Autodesk Inventor part; units mm, degrees
ref_plane "Work Plane1" through (60, 0, 0) normal (0, 0, 1) x (1, 0, 0)
ref_plane "YZ Plane" through (0, 0, 0) normal (1, 0, 0) x (0, 1, 0)
ref_plane "XZ Plane" through (0, 0, 0) normal (0, 1, 0) x (-1, 0, 0)
sketch "Sketch1" plane through (0, 0, 0) normal (0, 0, 1) x (1, 0, 0)
  line L0 (0, 3.175) -> (22.225, 3.175)
  line L1 (22.225, 3.175) -> (22.225, 0)
  line L2 (22.225, 0) -> (0, 0)
  line L3 (-4.445, 0) -> (26.67, 0)
  line L4 (0, -0.635) -> (0, 3.81)
  line L5 (0, 3.175) -> (0, 0)
  dimension "d1" = 6.35
  dimension "d52" = 22.225
revolve "Body" add sketch "Sketch1" angle 360 about axis through (22.225, 0, 0) along (-1, 0, 0)
sketch "Sketch2" plane through (0, 0, 0) normal (-1, 0, 0) x (0, 0, 1)
  line L0 (0, 5.4993) -> (4.7625, 2.7496)
  line L1 (4.7625, 2.7496) -> (4.7625, -2.7496)
  line L2 (4.7625, -2.7496) -> (0, -5.4993)
  line L3 (0, -5.4993) -> (-4.7625, -2.7496)
  line L4 (-4.7625, -2.7496) -> (-4.7625, 2.7496)
  line L5 (-4.7625, 2.7496) -> (0, 5.4993)
  line L6 (-6.6675, 0) -> (6.6675, 0)
  line L7 (0, 7.699) -> (0, -7.699)
  point P0 (0, 0)
  point P1 (0, 0)
  dimension "d10" = 9.525
extrude "Head" add sketch "Sketch2" along normal blind 4.826
sketch "Sketch3" plane through (0, 0, 0) normal (0, 0, 1) x (1, 0, 0)
  line L0 (-4.826, 0.9525) -> (-2.2606, 0.9525)
  line L1 (-2.2606, 0.9525) -> (-2.2606, -0.9525)
  line L2 (-2.2606, -0.9525) -> (-4.826, -0.9525)
  line L3 (-4.826, -0.9525) -> (-4.826, 0.9525)
  line L4 (-2.2606, 0) -> (-4.826, 0) construction
  line L5 (-5.3391, 0) -> (-1.7475, 0)
  line L6 (-4.826, 2.7496) -> (-4.826, -2.7496)
  dimension "d11" = 1.905
  dimension "d13" = 2.5654
extrude "Slot" cut sketch "Sketch3" along normal through all both and the other way through all
sketch "Sketch4" plane through (0, 0, 0) normal (0, 0, 1) x (1, 0, 0)
  line L0 (-4.826, 4.7625) -> (-4.826, 5.4993)
  line L1 (-4.826, 5.4993) -> (-4.4006, 5.4993)
  line L2 (-4.4006, 5.4993) -> (-4.826, 4.7625)
  line L3 (-4.4006, 5.4993) -> (-4.826, 5.4993)
  line L4 (-4.826, 5.4993) -> (-4.826, 4.7625)
  line L5 (-4.826, 5.4993) -> (-4.826, 2.7496)
  line L6 (-5.7912, 0) -> (0.9652, 0)
  line L7 (0, 5.4993) -> (-4.826, 5.4993)
  dimension "d4" = 30
  dimension "d17" = 9.525
revolve "Chamfer1" cut sketch "Sketch4" angle 360 about axis through (-10, 0, 0) along (1, 0, 0)
thread "Thread"
chamfer "Chamfer2" distance 0.635 distance2 0.6351 1 edges at (22.225, -3.175, 0) measured on face at (22.225, -0.1276, -1.0506)
ref_plane "Work Plane1" through (60, 0, 0) normal (0, 0, 1) x (1, 0, 0)
equation "\"d1\" = GD"
equation "\"d52\" = NLG"
equation "\"d10\" = SW"
equation "\"d2\" = KOH - SD"
equation "\"d11\" = SBR"
equation "\"d13\" = STI"
equation "\"d4\" = ANG1"
equation "\"d17\" = SW0"
equation "\"d15\" = GEL"
equation "\"d5\" = -0.5 * SPD + 0.5 * GD"
equation "\"NLG\" = 22.225"
equation "\"GD\" = NND"
equation "\"KOH\" = 4.826"
equation "\"GEL\" = 19.05"
equation "\"SW\" = 9.525"
equation "\"SW0\" = 9.525"
equation "\"SPD\" = GD1"
equation "\"SD2\" = NND"
equation "\"SD\" = 0"
equation "\"ANG1\" = 30deg"
equation "\"GUL\" = -0.5 * GD1 + 0.5 * NND"
equation "\"STI\" = 2.5654"
equation "\"SBR\" = 1.905"
equation "\"RR\" = 0.57912"
equation "\"THREADDIA\" = 6.35"
equation "\"TOA\" = 30deg"
equation "\"BDM\" = NND"
equation "\"FAWI\" = 45deg"
equation "\"NND\" = 6.35"
equation "\"E0\" = 1.155 * SW"
equation "\"GAL\" = 0.635"
equation "\"GD1\" = 5.08"
properties part number "ANSI B18.6.3 - 1/4-20x0.875, SHHMSI" material "Steel, Mild"
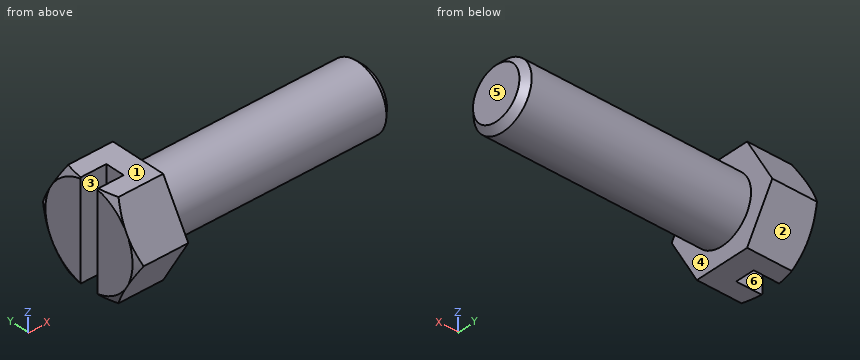
Work out the finished part from the listing and answer in its coordinate system (mm). Face numbers are marked on the shaded views. A direction names the side the tool comes from. Give positions to 0.01 mm unless a question says otherwise; leave off trailing zeros. Loops run counter-clockwise (first coordinate to the right, second up) from the corner with the lowest first, then second, coordinate; pieces in that order, holes last. Notation, with made-up numbers: (-33.75, -4.75) -> (-5.75, -4.75) arc R25 cw to (-5.75, 33.25) -> close; hole circle Ø10 at (-7.75, 29.5). An arc over 180 degrees is marked (long way). Use a Markdown table: item, result. Add a question column.
1. Determine the mould class of the marked faces 1, 2 and 3 for opening direction Y: released by +Y, released by -Y, zero draft, split by the parting line, or undercut.
2. Section A-A on y = 0 is taken. Determine the outline of the cut face in (x, z) (1 decimal).
3. Section B-B on x = 12.5 is taken. Determine the outline of the cut face in (y, z) (3 decimals), and give its area (3 significant figures).
4. Find the intervals of material crossed by probe 1 along X at (y, z) = (2, 2.5); probe 2 along X at (y, z) = (-0.75, 4); probe 3 along Y at (x, z) = (7.5, 0) (3 decimals), in increasing order.
5. For the marked faces 4, 5 and 6, determine the directions among +Z, -Z, +X, -X, +Y, -Y from which every point of the face is accessible in a straight line to the end or side of a thin tool.
6. Flat-ended cylindrical pins translate along their axes: pin 1 Ø0.8 at (x, z) = (-4, 0.5) entering from +Y; pin 2 Ø5 at (x, z) = (5.5, -1.5) entering from -Y (3 decimals); pin 3 Ø1.5 at (x, y) = (3.5, -2) entering from -Z; pin 4 Ø2 at (x, z) = (-4, 0.5) entering from -Y. Find the tip coordinate at first contact, or state that the pin passes through.
Results below:
| question | item | result |
|---|---|---|
| 1 | face 1 | zero draft |
| 1 | face 2 | released by +Y |
| 1 | face 3 | undercut |
| 2 | outline | (-2.3, -4.8) -> (0, -4.8) -> (0, -3.2) -> (21.6, -3.2) -> (22.2, -2.5) -> (22.2, 2.5) -> (21.6, 3.2) -> (0, 3.2) -> (0, 4.8) -> (-2.3, 4.8) -> close |
| 3 | outline | circle Ø6.35 at (0, 0) |
| 3 | area | 31.7 mm^2 |
| 4 | probe 1 | x = -4.83 to 0 |
| 4 | probe 2 | x = -2.26 to 0 |
| 4 | probe 3 | y = -3.175 to 3.175 |
| 5 | face 4 | +X |
| 5 | face 5 | +Z, -Z, +X, +Y, -Y |
| 5 | face 6 | +Z, -Z, -X |
| 6 | pin 1 | stops at y = 5.44 |
| 6 | pin 2 | stops at y = -3.175 |
| 6 | pin 3 | stops at z = -2.92 |
| 6 | pin 4 | stops at y = -5.5 |
